Geometry: final body of the model. Coordinates: model frame, mm. Coordinates: 2 decimals unless noted, no trailing zeros. Write each loop counter-clockwise with the first axis right and the second up, starting at its lowest first coordinate (ties: lowest second). Pieces come first, ordered by that corner, then holes. Notation, with made-up numbers: (64, 43.25) -> (109, 43.25) arc R26 cw to (109, 71.25) -> close; hole circle Ø6 at (34, 31). An arc over 180 degrees is marked (long way). One line per item, written item: value.
```python
from build123d import *

# Parameters (mm, degrees)
F0_W     = 177.8
F0_H     = 50.8
F0_R     = 2.5527
F0_R_2   = 14.2875
F1_DEPTH = 25.4
F2_W     = 22.225
F2_H     = 47.625
F3_DEPTH = 177.801
F4_R     = 2.5527
F5_DEPTH = 50.801


with BuildPart() as f1:
    # F0 (on Right) → F1 (new body)
    with BuildSketch(Plane.YZ):
        Rectangle(F0_W, F0_H)
        with Locations((-25.4, -12.7)):
            Circle(F0_R, mode=Mode.SUBTRACT)
        with Locations((-84.12223, -11.90625)):
            Circle(F0_R, mode=Mode.SUBTRACT)
        with Locations((-63.5, 0)):
            Circle(F0_R_2, mode=Mode.SUBTRACT)
        with Locations((-42.87777, -11.90625)):
            Circle(F0_R, mode=Mode.SUBTRACT)
        with Locations((0, -12.7)):
            Circle(F0_R, mode=Mode.SUBTRACT)
        with Locations((25.4, -12.7)):
            Circle(F0_R, mode=Mode.SUBTRACT)
        with Locations((50.8, -12.7)):
            Circle(F0_R, mode=Mode.SUBTRACT)
        with Locations((76.2, -12.7)):
            Circle(F0_R, mode=Mode.SUBTRACT)
        with Locations((-84.12223, 11.90625)):
            Circle(F0_R, mode=Mode.SUBTRACT)
        with Locations((-42.87777, 11.90625)):
            Circle(F0_R, mode=Mode.SUBTRACT)
        with Locations((-25.4, 12.7)):
            Circle(F0_R, mode=Mode.SUBTRACT)
        with Locations((0, 12.7)):
            Circle(F0_R, mode=Mode.SUBTRACT)
        with Locations((25.4, 12.7)):
            Circle(F0_R, mode=Mode.SUBTRACT)
        with Locations((50.8, 12.7)):
            Circle(F0_R, mode=Mode.SUBTRACT)
        with Locations((76.2, 12.7)):
            Circle(F0_R, mode=Mode.SUBTRACT)
    extrude(amount=F1_DEPTH)

    # F2 (on face) → F3 (cut, through all)
    with BuildSketch(Plane.XZ.offset(88.9)):
        with Locations((12.7, 0)):
            Rectangle(F2_W, F2_H)
    extrude(amount=-F3_DEPTH, mode=Mode.SUBTRACT)

    # F4 (on face) → F5 (cut, through all)
    with BuildSketch(Plane.XY.offset(25.4)):
        with Locations((12.7, 76.2)):
            Circle(F4_R)
        with Locations((12.7, 50.8)):
            Circle(F4_R)
        with Locations((12.7, 25.4)):
            Circle(F4_R)
        with Locations((12.7, 0)):
            Circle(F4_R)
        with Locations((12.7, -25.4)):
            Circle(F4_R)
        with Locations((12.7, -50.8)):
            Circle(F4_R)
        with Locations((12.7, -76.2)):
            Circle(F4_R)
        with Locations((12.7, -101.6)):
            Circle(F4_R)
        with Locations((12.7, -127)):
            Circle(F4_R)
    extrude(amount=-F5_DEPTH, mode=Mode.SUBTRACT)


solid = f1.part
```
(1) Section C-C (y = 50.8). State how many separate pieces and enclosed holes the cut face has, then the cut area to 3 significant figures.
Responses:
separate pieces: 6
enclosed holes: 0
area: 183 mm2
(2) Line query: line 1 (Z direction, x = 23.75, y = 60); line 2 (X direction, y = 28, z = -3.5); line 3 (Z direction, x = 25, y = 25.4). Output: solid intervals per line, ascending. Write a range as [from, to].
Responses:
line 1: z = [-25.4, -23.81], [23.81, 25.4]
line 2: x = [0, 1.59], [23.81, 25.4]
line 3: z = [-25.4, -15.25], [-10.15, 10.15], [15.25, 25.4]
(3) Section D-D (x = 19.5). Return the cut outline in (y, z).
Responses:
outline: (-88.9, -25.4) -> (88.9, -25.4) -> (88.9, -23.81) -> (-88.9, -23.81) -> close; (-88.9, 23.81) -> (88.9, 23.81) -> (88.9, 25.4) -> (-88.9, 25.4) -> close
(4) Section A-A (y = -63.5). Return the cut outline in (x, z).
Responses:
outline: (0, -25.4) -> (25.4, -25.4) -> (25.4, -14.29) -> (23.81, -14.29) -> (23.81, -23.81) -> (1.59, -23.81) -> (1.59, -14.29) -> (0, -14.29) -> close; (0, 14.29) -> (1.59, 14.29) -> (1.59, 23.81) -> (23.81, 23.81) -> (23.81, 14.29) -> (25.4, 14.29) -> (25.4, 25.4) -> (0, 25.4) -> close
(5) Pull-direction query (Z, two-part tool) for faces 1 (the flat face through (15.3, -1.2, -25.4)), 2 (the flat face through (0, -1, 0)), 3 (the cylindrical face through (0.783, -86.148, 10.353)); classes: released by +Z, released by -Z, zero draft, split by the parting line, or undercut.
Responses:
face 1: released by -Z
face 2: zero draft
face 3: undercut
(6) First-contact query: pin 1 (3 mm diameter, centred on y = -42.88, z = -11.91, fed in from -X); pin 2 (8 mm diameter, centred on y = 0, z = 12.7, fed in from -X). Flat tips, straight axial feed; report the tip coordinate or a pass-through.
Responses:
pin 1: passes through
pin 2: stops at x = 0
(7) Section B-B (z = 21). Return the cut outline in (x, y).
Responses:
outline: (0, -88.9) -> (1.59, -88.9) -> (1.59, 88.9) -> (0, 88.9) -> close; (23.81, -88.9) -> (25.4, -88.9) -> (25.4, 88.9) -> (23.81, 88.9) -> close
